from build123d import *

# Parameters (mm, degrees)
F1_DEPTH = 3.81
F3_DEPTH = 7.62
F5_DEPTH = 11.431
F7_DEPTH = 4.63296


with BuildPart() as f1:
    # F0 (on Front) → F1 (new body)
    with BuildSketch(Plane.XZ):
        with BuildLine():
            ThreePointArc((-26.9875, -2.54), (-22.1518329574, -14.2143329574), (-10.4775, -19.05))
            Line((-10.4775, -19.05), (10.4775, -19.05))
            ThreePointArc((10.4775, -19.05), (22.1518329574, -14.2143329574), (26.9875, -2.54))
            Line((26.9875, -2.54), (26.9875, 2.54))
            ThreePointArc((26.9875, 2.54), (22.1518329574, 14.2143329574), (10.4775, 19.05))
            Line((10.4775, 19.05), (-10.4775, 19.05))
            ThreePointArc((-10.4775, 19.05), (-22.1518329574, 14.2143329574), (-26.9875, 2.54))
            Line((-26.9875, 2.54), (-26.9875, -2.54))
        make_face()
    extrude(amount=F1_DEPTH)

    # F2 (on face) → F3 (join)
    with BuildSketch(Plane.XZ.offset(3.81)):
        with BuildLine():
            ThreePointArc((-22.225, -3.556), (-19.1748100193, -10.9198100193), (-11.811, -13.97))
            Line((-11.811, -13.97), (11.811, -13.97))
            ThreePointArc((11.811, -13.97), (19.1748100193, -10.9198100193), (22.225, -3.556))
            Line((22.225, -3.556), (22.225, 3.556))
            ThreePointArc((22.225, 3.556), (19.1748100193, 10.9198100193), (11.811, 13.97))
            Line((11.811, 13.97), (-11.811, 13.97))
            ThreePointArc((-11.811, 13.97), (-19.1748100193, 10.9198100193), (-22.225, 3.556))
            Line((-22.225, 3.556), (-22.225, -3.556))
        make_face()
    extrude(amount=F3_DEPTH)

    # F4 (on face) → F5 (cut, through all)
    with BuildSketch(Plane.XZ.offset(11.43)):
        with BuildLine():
            ThreePointArc((-14.2494, -3.7719), (-13.5054512242, -5.5679512242), (-11.7094, -6.3119))
            Line((-11.7094, -6.3119), (11.7094, -6.3119))
            ThreePointArc((11.7094, -6.3119), (13.5054512242, -5.5679512242), (14.2494, -3.7719))
            Line((14.2494, -3.7719), (14.2494, 3.7719))
            ThreePointArc((14.2494, 3.7719), (13.5054512242, 5.5679512242), (11.7094, 6.3119))
            Line((11.7094, 6.3119), (-11.7094, 6.3119))
            ThreePointArc((-11.7094, 6.3119), (-13.5054512242, 5.5679512242), (-14.2494, 3.7719))
            Line((-14.2494, 3.7719), (-14.2494, -3.7719))
        make_face()
    extrude(amount=-F5_DEPTH, mode=Mode.SUBTRACT)

    # F6 (on face) → F7 (cut)
    with BuildSketch(Plane.XZ.offset(11.43)):
        with BuildLine():
            Line((11.4554, 11.6459), (-11.4554, 11.6459))
            ThreePointArc((-11.4554, 11.6459), (-17.2027639175, 9.2652639175), (-19.5834, 3.5179))
            Line((-19.5834, 3.5179), (-19.5834, -3.5179))
            ThreePointArc((-19.5834, -3.5179), (-17.2027639175, -9.2652639175), (-11.4554, -11.6459))
            Line((-11.4554, -11.6459), (11.4554, -11.6459))
            ThreePointArc((11.4554, -11.6459), (17.2027639175, -9.2652639175), (19.5834, -3.5179))
            Line((19.5834, -3.5179), (19.5834, 3.5179))
            ThreePointArc((19.5834, 3.5179), (17.2027639175, 9.2652639175), (11.4554, 11.6459))
        make_face()
        with BuildLine():
            Line((11.4554, -7.5819), (-11.4554, -7.5819))
            ThreePointArc((-11.4554, -7.5819), (-14.3290819587, -6.3915819587), (-15.5194, -3.5179))
            Line((-15.5194, -3.5179), (-15.5194, 3.5179))
            ThreePointArc((-15.5194, 3.5179), (-14.3290819587, 6.3915819587), (-11.4554, 7.5819))
            Line((-11.4554, 7.5819), (11.4554, 7.5819))
            ThreePointArc((11.4554, 7.5819), (14.3290819587, 6.3915819587), (15.5194, 3.5179))
            Line((15.5194, 3.5179), (15.5194, -3.5179))
            ThreePointArc((15.5194, -3.5179), (14.3290819587, -6.3915819587), (11.4554, -7.5819))
        make_face(mode=Mode.SUBTRACT)
    extrude(amount=-F7_DEPTH, mode=Mode.SUBTRACT)


solid = f1.part
The listing builds one solid part. Answer for the finished solid, in the listing's coordinates (mm). A direction names the side the tool comes from. Give positions to 0.01 mm unless a question says otherwise; leave off trailing zeros. Write each loop counter-clockwise with the first axis right and the second up, starting at its lowest first coordinate (ties: lowest second). Pieces come first, ordered by that corner, then holes.
1) Section B-B (x = 4.5) is taken. Write down the section's boundary in (y, z).
2) Given P1, Ø3, axis at x = 13.5, y = -9, coming from the +Z side; P2, Ø1.4, axis at y = -9.5, z = 1, coming from the +X side (3 decimals); P3, Ø3.5, axis at x = 3, y = -9, coming from the -Z side, each flat-ended and moving along its own axis, determine where each tip first touches the part or whether it passes through.
3) For a pull along X with two mould halves and no side action, classify faces 1 (the face through (19.583, -9, 0)), 2 (the face through (0, -6, -6.312)), 3 (the face through (-19.255, -7.567, -10.838)), 4 (the face through (22.023, -1.878, -14.342)) as pulls with the +X half, pulls with the -X half, needs draft (parallel to the pull), parting line crosses it, or undercut.
4) Find the intervals of material crossed by L1, parallel to Z at x = -7, y = -11; L2, parallel to Z at x = -11, y = -1.25; L3, parallel to Z at x = 4, y = -5, in increasing order.
5) Section A-A (y = -8.25) is taken. Count the separate pieces of the cut face and the enclosed holes in it, and give its area (3 significant figures).
6) A tool of negligible diameter and unlimited length cuts with its end or side. For faces 5 (the face through (0, -9, -11.646)), 6 (the face through (22.225, -8, 0)), 7 (the face through (-13.525, -5.795, -5.548)), 8 (the face through (-19.093, -7.567, 11)), from which of +Z, -Z, +X, -X, +Y, -Y can it reach the whole face along a straight path? Write none if from no direction.
7) Section D-D (y = -2.25) is taken. Write down the section's boundary in (x, z), and give its area (3 significant figures).
8) Section C-C (z = -4.5) is taken. Write down the section's boundary in (x, y).
Response:
1. outline: (-11.43, -13.97) - (-3.81, -13.97) - (-3.81, -19.05) - (0, -19.05) - (0, -6.31) - (-11.43, -6.31) - (-11.43, -7.58) - (-6.8, -7.58) - (-6.8, -11.65) - (-11.43, -11.65) - close; (-11.43, 6.31) - (0, 6.31) - (0, 19.05) - (-3.81, 19.05) - (-3.81, 13.97) - (-11.43, 13.97) - (-11.43, 11.65) - (-6.8, 11.65) - (-6.8, 7.58) - (-11.43, 7.58) - close
2. P1: stops at z = 13.97
2. P2: stops at x = 22.225
2. P3: stops at z = -13.97
3. face 1: undercut
3. face 2: undercut
3. face 3: pulls with the -X half
3. face 4: pulls with the +X half
4. L1: z = -13.97 to -11.65, -7.58 to -6.31, 6.31 to 7.58, 11.65 to 13.97
4. L2: z = -19.04 to -6.31, 6.31 to 19.04
4. L3: z = -13.97 to -6.31, 6.31 to 13.97
5. separate pieces: 2
5. enclosed holes: 2
5. area: 396 mm2
6. face 5: -Y
6. face 6: +Z, -Z, +X, -Y
6. face 7: +Y, -Y
6. face 8: +Z, -X, -Y
7. outline: (-26.99, -2.54) arc R16.51 ccw to (-10.48, -19.05) - (10.48, -19.05) arc R16.51 ccw to (26.99, -2.54) - (26.99, 2.54) arc R16.51 ccw to (10.48, 19.05) - (-10.48, 19.05) arc R16.51 ccw to (-26.99, 2.54) - close; hole (-14.25, -3.77) arc R2.54 ccw to (-11.71, -6.31) - (11.71, -6.31) arc R2.54 ccw to (14.25, -3.77) - (14.25, 3.77) arc R2.54 ccw to (11.71, 6.31) - (-11.71, 6.31) arc R2.54 ccw to (-14.25, 3.77) - close
7. area: 1,470 mm2
8. outline: (-26.87, -3.81) - (-22.18, -3.81) - (-22.18, -11.43) - (-19.52, -11.43) - (-19.52, -6.8) - (-15.4, -6.8) - (-15.4, -11.43) - (-14.14, -11.43) - (-14.14, 0) - (-26.87, 0) - close; (14.14, -11.43) - (15.4, -11.43) - (15.4, -6.8) - (19.52, -6.8) - (19.52, -11.43) - (22.18, -11.43) - (22.18, -3.81) - (26.87, -3.81) - (26.87, 0) - (14.14, 0) - close
